```python
from build123d import *

# Parameters (mm, degrees)
SKETCH_W     = 100
SKETCH_H     = 6
PAD_DEPTH    = 1
CHAMFER_SIZE = 1
PAD001_DEPTH = 3


with BuildPart() as chamfer_body:
    # Sketch → Pad (new body)
    with BuildSketch(Plane.XY):
        Rectangle(SKETCH_W, SKETCH_H)
    extrude(amount=PAD_DEPTH)

    # Chamfer
    chamfer_edges = [chamfer_body.edges().sort_by_distance(p)[0] for p in [
        (-50, 3, 0.5),
        (-50, -3, 0.5),
        (50, 3, 0.5),
        (50, -3, 0.5),
    ]]
    chamfer(chamfer_edges, length=CHAMFER_SIZE)


with BuildPart() as fusion:
    # Sketch001 → Pad001 (new body, symmetric)
    with BuildSketch(Plane.XZ):
        Polygon((-50, 8), (-50, 6.5), (-43.5, 0), (43.5, 0), (50, 6.5), (50, 8), align=None)
        Polygon((-42.5, 1), (-48, 6.5), (-17.333333, 6.5), (-15.5, 1), align=None, mode=Mode.SUBTRACT)
        Polygon((48, 6.5), (42.5, 1), (15.5, 1), (17.333333, 6.5), align=None, mode=Mode.SUBTRACT)
        Polygon((-13.5, 1), (-15.333333, 6.5), (15.333333, 6.5), (13.5, 1), align=None, mode=Mode.SUBTRACT)
    extrude(amount=PAD001_DEPTH, both=True)

    # Fusion: union Chamfer body
    add(chamfer_body.part)


solid = fusion.part
```
For this review, take the finished solid that the model builds, in its own axes (mm). A direction names the side the tool comes from. Coordinates: 2 decimals unless noted, no trailing zeros. Order: outer loops, then holes, each group sorted by start corner. A loop starts at its lowest first (then second) coordinate and runs counter-clockwise, first axis right, second up. Notation, with made-up numbers: (80.25, 34.5) -> (110.25, 34.5) arc R16 ccw to (110.25, 48.5) -> close; hole circle Ø7 at (57.25, -32). An arc over 180 degrees is marked (long way). Use CSV: the item, a comma, the result in double quotes. Start each with the question number.
Item 1: For faces 1 (the face through (47.2, 0, 3.7)), 2 (the face through (-47.3, 0, 3.8)), 3 (the face through (16.4, 0, 3.7)), list the 3-axis set-ups (+Z, -Z, +X, -X, +Y, -Y) from which the entire face can be reached by the end or side of a thin tool; tool diameter is ignored.
Item 2: We need section A-A, the plane x = 34.5. Give the boundary of the cut face in (y, z), then the cut area to 3 significant figures.
Item 3: Draft analysis for pull direction Z (two halves, no side actions). For faces 4 (the face through (1, 0, 8)), 5 (the face through (-1, 0, 0)), 6 (the face through (32, 0, 6.5)), state which applies: pulls with the +Z half, pulls with the -Z half, needs draft (parallel to the pull), parting line crosses it, or undercut.
Item 4: We need section C-C, the plane z = 3.5. Give the boundary of the cut face in (x, y).
Item 5: Insertion check: pin 1 (1.5 mm diameter, centred on y = -2, z = 3.5, fed in from +X); pin 2 (3 mm diameter, centred on x = 26.5, y = 0.5, fed in from -Z). Each pin has a flat end and moves straight along its axis. Give the tip position at first contact, or say it passes through.
Item 6: Wall thickness on probe 1 along Z at (x, y) = (-1.5, -1.5); probe 2 along X at (y, z) = (-0.25, 1.25); probe 3 along X at (y, z) = (0.5, 3.25): over which ranges is each line inside the solid? List them lowest first.
Item 7: We need section B-B, the plane y = -0.25. Give the boundary of the cut face in (x, z), then the cut area to 3 significant figures.
Derived:
1,face 1,"+X, +Y, -Y"
1,face 2,"-X, +Y, -Y"
1,face 3,"+Y, -Y"
2,outline,"(-3, 0) -> (3, 0) -> (3, 1) -> (-3, 1) -> close; (-3, 6.5) -> (3, 6.5) -> (3, 8) -> (-3, 8) -> close"
2,area,"15.0 mm^2"
3,face 4,"pulls with the +Z half"
3,face 5,"pulls with the -Z half"
3,face 6,"undercut"
4,outline,"(-47, -3) -> (-45, -3) -> (-45, 3) -> (-47, 3) -> close; (-16.33, -3) -> (-14.33, -3) -> (-14.33, 3) -> (-16.33, 3) -> close; (14.33, -3) -> (16.33, -3) -> (16.33, 3) -> (14.33, 3) -> close; (45, -3) -> (47, -3) -> (47, 3) -> (45, 3) -> close"
5,pin 1,"stops at x = 47.75"
5,pin 2,"stops at z = 0"
6,probe 1,"z = 0 to 1, 6.5 to 8"
6,probe 2,"x = -44.75 to -42.75, -15.58 to -13.58, 13.58 to 15.58, 42.75 to 44.75"
6,probe 3,"x = -46.75 to -44.75, -16.25 to -14.25, 14.25 to 16.25, 44.75 to 46.75"
7,outline,"(-50, 0) -> (50, 0) -> (50, 1) -> (44.5, 1) -> (50, 6.5) -> (50, 8) -> (-50, 8) -> (-50, 6.5) -> (-44.5, 1) -> (-50, 1) -> close; hole (-48, 6.5) -> (-42.5, 1) -> (-15.5, 1) -> (-17.33, 6.5) -> close; hole (-15.33, 6.5) -> (-13.5, 1) -> (13.5, 1) -> (15.33, 6.5) -> close; hole (15.5, 1) -> (42.5, 1) -> (48, 6.5) -> (17.33, 6.5) -> close"
7,area,"294 mm^2"
